Here's the drawing with two shaded views (mm, measured from the low corner). I have some questions. Round coordinates to 2 decimals unless told otherwise and drop trailing zeros. Write each loop counter-clockwise with the first axis right and the second up, starting at its lowest first coordinate (ties: lowest second). Pieces come first, ordered by that corner, then holes. Notation, with made-up numbers: (18, 2) - (26, 2) arc R27 ccw to (26, 32) - close; hole circle Ø8 at (11, -25). An arc over 180 degrees is marked (long way). Return JSON: item names as keys, results as strings. Group by question number.
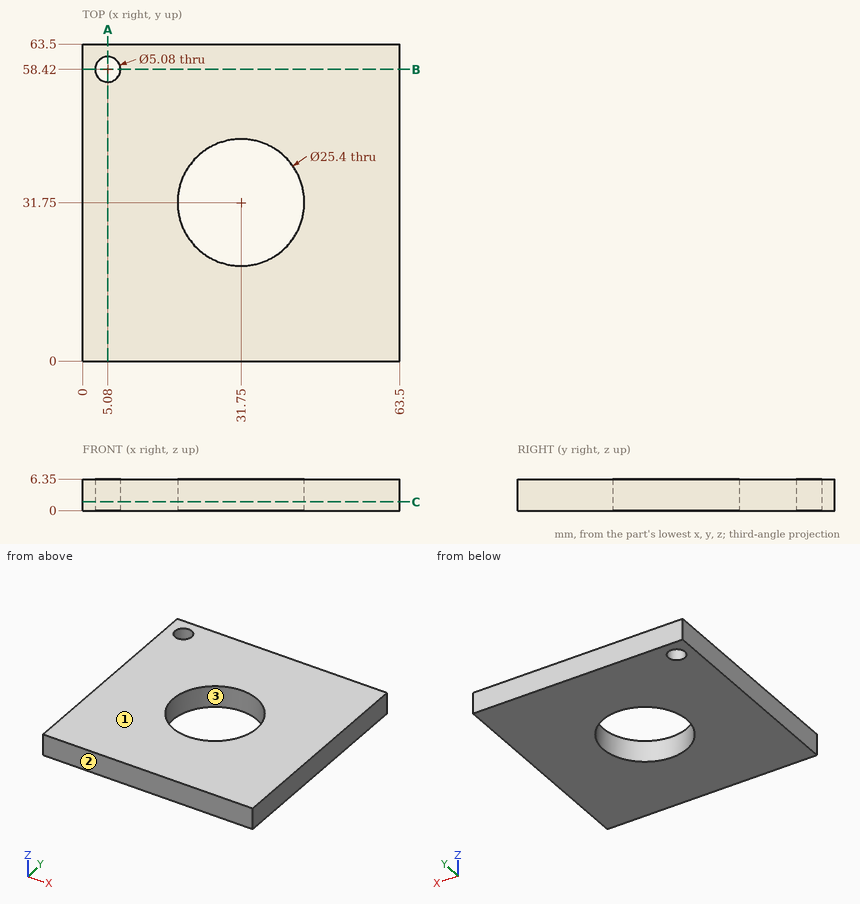
1) Imagine slicing it at C-C (z = 1.75). Please give me the cut outline in (x, y), plus the area to 3 significant figures.
2) Imagine slicing it at B-B (y = 58.42). Please give me the cut outline in (x, z).
3) Will this pin go through, and if not, where does the flat tip stop? pin 1 Ø5 at (x, y) = (39.5, 11) entering from -Z.
4) If we mould it in two halves opening along Y, with no side actions, what happens to the marked faces 1, 2 and 3? For each: released by +Y, released by -Y, zero draft, split by the parting line, or undercut.
5) I need wall thicknesses on line 1 along Y through (x, z) = (5.08, 3); line 2 along Y through (x, z) = (31.75, 4.75). Which ranges of each line are inside material? Lowest first, please.
6) Imagine slicing it at A-A (x = 5.08). Please give me the cut outline in (y, z), plus the area to 3 significant figures.
Results found:
{
 "1": {"outline": "(0, 0) - (63.5, 0) - (63.5, 63.5) - (0, 63.5) - close; hole circle Ø5.08 at (5.08, 58.42); hole circle Ø25.4 at (31.75, 31.75)", "area": "3,510 mm²"},
 "2": {"outline": "(0, 0) - (2.54, 0) - (2.54, 6.35) - (0, 6.35) - close; (7.62, 0) - (63.5, 0) - (63.5, 6.35) - (7.62, 6.35) - close"},
 "3": {"pin 1": "stops at z = 0"},
 "4": {"face 1": "zero draft", "face 2": "released by -Y", "face 3": "undercut"},
 "5": {"line 1": "y = 0 to 55.88, 60.96 to 63.5", "line 2": "y = 0 to 19.05, 44.45 to 63.5"},
 "6": {"outline": "(0, 0) - (55.88, 0) - (55.88, 6.35) - (0, 6.35) - close; (60.96, 0) - (63.5, 0) - (63.5, 6.35) - (60.96, 6.35) - close", "area": "371 mm²"}
}
